```python
from build123d import *

# Parameters (mm, degrees)
BOSS_EXTRUDE1_DEPTH = 10.16
SKETCH2_R           = 1.5
CUT_EXTRUDE1_DEPTH  = 32.4325
SKETCH3_R           = 1.5
CUT_EXTRUDE2_DEPTH  = 7.35
SKETCH4_W           = 12.726748703
SKETCH4_H           = 1.27
CUT_EXTRUDE3_DEPTH  = 11.16


with BuildPart() as part:
    # Sketch1 → Boss-Extrude1 (new body)
    with BuildSketch(Plane(origin=(0, 0, 0), x_dir=(1, 0, 0), z_dir=(0, 1, 0))):
        with BuildLine():
            Line((0, 0), (-12.7, 0))
            ThreePointArc((-12.7, 0), (-40.313380236, -30.054590243), (-72.594133091, -5.08))
            Line((-72.594133091, -5.08), (-83.889837791, -5.08))
            Line((-83.889837791, -5.08), (-83.889837791, -11.43))
            Line((-83.889837791, -11.43), (-77.539837791, -11.43))
            ThreePointArc((-77.539837791, -11.43), (-40.243263553, -36.418432925), (-6.906413502, -6.35))
            Line((-6.906413502, -6.35), (0, -6.35))
            Line((0, -6.35), (0, 0))
        make_face()
    extrude(amount=BOSS_EXTRUDE1_DEPTH)

    # Sketch2 → Cut-Extrude1 (cut, through all)
    with BuildSketch(Plane(origin=(0, 0, 5.08), x_dir=(-1, 0, 0), z_dir=(0, 0, -1))):
        with Locations((80.714837791, 7.62)):
            Circle(SKETCH2_R)
        with Locations((80.714837791, 2.54)):
            Circle(SKETCH2_R)
    extrude(amount=-CUT_EXTRUDE1_DEPTH, mode=Mode.SUBTRACT)

    # Sketch3 → Cut-Extrude2 (cut, through all)
    with BuildSketch(Plane.XY.offset(6.35)):
        with Locations((-3.453206751, 5.08)):
            Circle(SKETCH3_R)
    extrude(amount=-CUT_EXTRUDE2_DEPTH, mode=Mode.SUBTRACT)

    # Sketch4 → Cut-Extrude3 (cut, through all)
    with BuildSketch(Plane.XZ):
        with Locations((-6.363374352, 0.635)):
            Rectangle(SKETCH4_W, SKETCH4_H)
    extrude(amount=-CUT_EXTRUDE3_DEPTH, mode=Mode.SUBTRACT)


solid = part.part
```
Read the model definition and answer for the solid it produces. Units are mm, in the model's axes. A direction names the side the tool comes from. Coordinates: 2 decimals unless noted, no trailing zeros. Write each loop counter-clockwise with the first axis right and the second up, starting at its lowest first coordinate (ties: lowest second). Pieces come first, ordered by that corner, then holes. Notation, with made-up numbers: (-21.5, 35.25) -> (1.5, 35.25) arc R19 ccw to (1.5, 52.25) -> close; hole circle Ø7 at (33, 57.5). An arc over 180 degrees is marked (long way). Write item = value, one per line.
(1) Which of the six approach directions +Z, -Z, +X, -X, +Y, -Y give full straight-line access (tool end or side, diameter ignored) to faces 1 (the face through (-81, 5, 11.43)), 2 (the face through (-78, 5, 5.08)), 3 (the face through (-6, 5, 1.27))?
From the geometry:
face_1 = +Z, -X, +Y, -Y
face_2 = -Z, -X, +Y, -Y
face_3 = -Z, +X, -X, +Y, -Y
(2) Section C-C on x = -35.5 is taken. Write down the section's boundary in (y, z).
From the geometry:
outline = (0, 29.25) -> (10.16, 29.25) -> (10.16, 35.76) -> (0, 35.76) -> close
(3) Section B-B on z = 23 is taken. Write down the section's boundary in (x, y), plus the area to 3 significant figures.
From the geometry:
outline = (-71.22, 0) -> (-62.38, 0) -> (-62.38, 10.16) -> (-71.22, 10.16) -> close; (-23.35, 0) -> (-14.5, 0) -> (-14.5, 10.16) -> (-23.35, 10.16) -> close
area = 180 mm2
(4) For a pull along Y with two mould halves and no side action, classify faces 4 (the face through (-79.609, 3.554, 8.211)), 5 (the face through (-3.778, 3.616, 3.846)), 6 (the face through (-42, 0, 31)), 7 (the face through (-5, 4, 6.35)) as +Y half, -Y half, draft (parallel to the pull), parting line (faces both ways), or undercut.
From the geometry:
face_4 = undercut
face_5 = undercut
face_6 = -Y half
face_7 = draft
(5) Section D-D on z = 29 is taken. Write down the section's boundary in (x, y), plus the area to 3 significant figures.
From the geometry:
outline = (-65.05, 0) -> (-51.16, 0) -> (-51.16, 10.16) -> (-65.05, 10.16) -> close; (-34.57, 0) -> (-20.68, 0) -> (-20.68, 10.16) -> (-34.57, 10.16) -> close
area = 282 mm2
(6) Given pin 1 Ø1.5 at (y, z) = (2, 12.5) entering from +X; pin 2 Ø3 at (x, y) = (-77.5, 6.5) entering from -Z; pin 3 Ø4 at (x, y) = (-80.71, 2.54) entering from +Z, each flat-ended and moving along its own axis, determine where each tip first touches the part or whether it passes through.
From the geometry:
pin_1 = -8.29
pin_2 = 5.08
pin_3 = 11.43
(7) Straight lines are drawn through the part: L1, parallel to X at y = 9.75, z = 13.5; L2, parallel to X at y = 9.75, z = 7; L3, parallel to Z at x = -39.5, y = 5. For each, find the intervals that lie inside material, in ascending order. Write a range as from..to.
From the geometry:
L1 = -76.79..-69.84, -15.89..-8.94
L2 = -83.89..-72.2, -13.52..-7.03
L3 = 29.97..36.36
